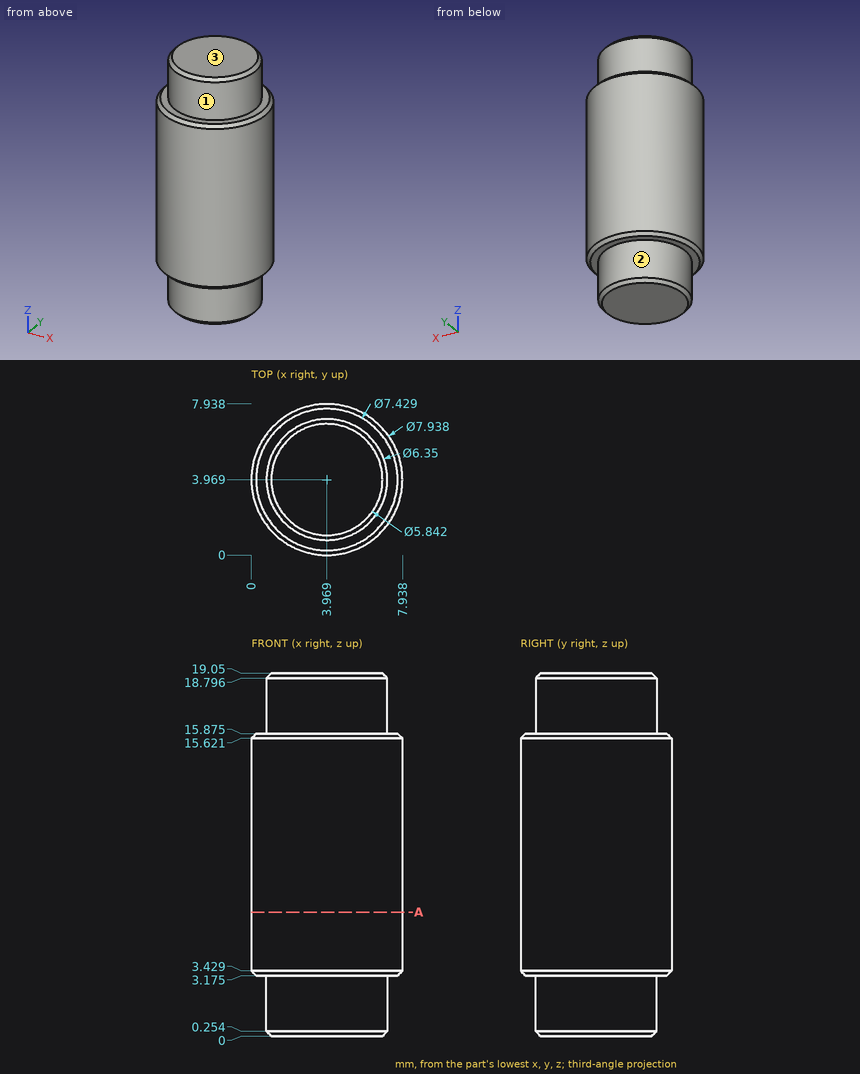
Here's the drawing with two shaded views (mm, measured from the low corner). I have some questions. A direction names the side the tool comes from. Coordinates: 2 decimals unless noted, no trailing zeros. Order: outer loops, then holes, each group sorted by start corner. A loop starts at its lowest first (then second) coordinate and runs counter-clockwise, first axis right, second up.
Q1. Please list where these lines run through material, in increasing order: L1, parallel to Z at x = 5, y = 7.5 (1 decimal); L2, parallel to X at y = 2.75, z = 7.5 (1 decimal); L3, parallel to X at y = 5.5, z = 9.
Q2. Will these pins go through, and if not, where does the flat tip stop? pin 1 (2 mm diameter, centred on x = 4.5, z = 17, fed in from -Y); pin 2 (3 mm diameter, centred on x = 2, z = 12, fed in from -Y).
Q3. Which directions (+Z, -Z, +X, -X, +Y, -Y) give clear straight access to the entire face, cutting with the end or side of a thin tool? Please do the marked faces 1, 2 and 3.
Q4. Suppose I cut it at A-A on z = 6.5. Please give me the cut outline in (x, y).
Answer:
1. L1: z = 3.2 to 15.9
1. L2: x = 0.2 to 7.7
1. L3: x = 0.31 to 7.63
2. pin 1: stops at y = 0.79
2. pin 2: stops at y = 0.03
3. face 1: +Z
3. face 2: -Z
3. face 3: +Z, +X, -X, +Y, -Y
4. outline: circle Ø7.94 at (3.97, 3.97)
